Job drawing, mm, ordinate dimensions from the low corner. One solid piece. Give positions to 0.01 mm unless a question says otherwise; leave off trailing zeros. Loops run counter-clockwise (first coordinate to the right, second up) from the corner with the lowest first, then second, coordinate; pieces in that order, holes last. Notation, with made-up numbers: M 11,-8.5 L 50,-8.5 A30 ccw 50,18.5 Z; hole C 26,80 d7. An arc over 180 degrees is marked long. Put each result on its own line as item: value.
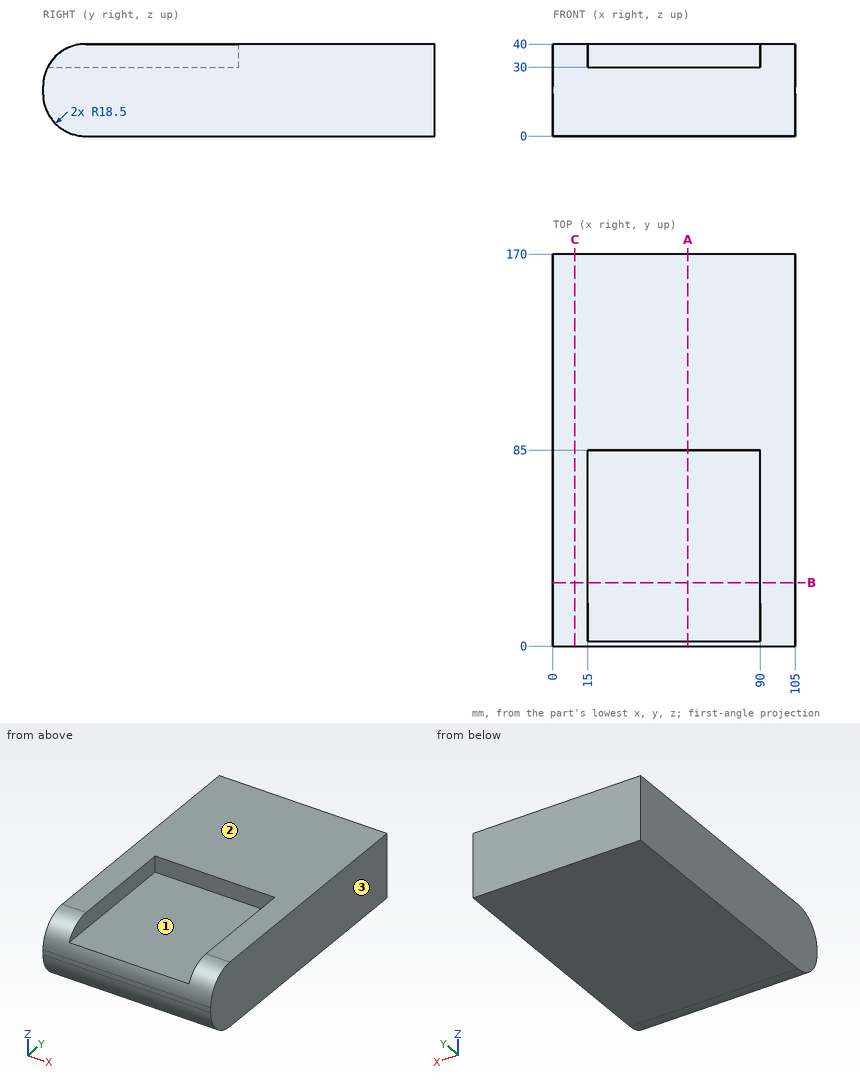
Q1. Drop flat-ended pins along their axis: pin 1 Ø8 at (x, z) = (38.5, 34.5) entering from -Y; pin 2 Ø10 at (x, y) = (28.5, 37.5) entering from +Z. Give the stop position or say it passes through.
Here are the results:
pin 1: y = 85
pin 2: z = 30
Q2. Slice it at C-C (x = 9.5). List the corners of the cut face in (y, z).
Here are the results:
outline: M 0,18.5 A18.5 ccw 18.5,0 L 170,0 L 170,40 L 18.5,40 A18.5 ccw 0,21.5 Z
Q3. Slice it at B-B (y = 27.5). List the corners of the cut face in (x, z).
Here are the results:
outline: M 0,0 L 105,0 L 105,40 L 90,40 L 90,30 L 15,30 L 15,40 L 0,40 Z
Q4. Mould opens along X. For the marked faces 1, 2 and 3 say: pulls with the +X half, pulls with the -X half, needs draft (parallel to the pull), parting line crosses it, or undercut.
Here are the results:
face 1: undercut
face 2: needs draft
face 3: pulls with the +X half
Q5. Slice it at A-A (x = 58.5). List the corners of the cut face in (y, z), and give its area (3 significant figures).
Here are the results:
outline: M 0,18.5 A18.5 ccw 18.5,0 L 170,0 L 170,40 L 85,40 L 85,30 L 2.07,30 A18.5 ccw 0,21.5 Z
area: 5,870 mm²
Q6. Probe line 1 (Z direction, x = 26, y = 82); line 2 (Y direction, x = 26, z = 32.5); line 3 (Y direction, x = 36, z = 10). List the from-to ranges inside material, lowest first. Write a range as from..to.
Here are the results:
line 1: 0..30
line 2: 85..170
line 3: 2.07..170
